```python
from build123d import *

# Parameters (mm, degrees)
SKETCH_1_W          = 70
SKETCH_1_H          = 70
EXTRUDE_1_DEPTH     = 3
CHAMFER_1_SIZE      = 6
SKETCH_2_R          = 2.1
CUT_EXTRUDE_1_DEPTH = 50.588305073
SKETCH_3_R          = 5.55
CUT_EXTRUDE_2_DEPTH = 50.588305073


with BuildPart() as part:
    # 草圖1 → 填料-伸長1 (new body)
    with BuildSketch(Plane.XY):
        Rectangle(SKETCH_1_W, SKETCH_1_H)
    extrude(amount=EXTRUDE_1_DEPTH)

    # 導角1
    chamfer_1_edges = [part.edges().sort_by_distance(p)[0] for p in [
        (-35, 35, 1.5),
        (35, 35, 1.5),
        (35, -35, 1.5),
        (-35, -35, 1.5),
    ]]
    chamfer(chamfer_1_edges, length=CHAMFER_1_SIZE)

    # 草圖2 → 除料-伸長1 (cut, through all)
    with BuildSketch(Plane(origin=(0, 0, 0), x_dir=(-1, 0, 0), z_dir=(0, 0, -1))):
        with Locations((0, 30)):
            Circle(SKETCH_2_R)
        with Locations((-30, -25)):
            Circle(SKETCH_2_R)
        with Locations((30, -25)):
            Circle(SKETCH_2_R)
    extrude(amount=-CUT_EXTRUDE_1_DEPTH, mode=Mode.SUBTRACT)

    # 草圖3 → 除料-伸長2 (cut, through all)
    with BuildSketch(Plane(origin=(0, 0, 0), x_dir=(-1, 0, 0), z_dir=(0, 0, -1))):
        with Locations((-17, 15)):
            Circle(SKETCH_3_R)
    extrude(amount=-CUT_EXTRUDE_2_DEPTH, mode=Mode.SUBTRACT)


solid = part.part
```
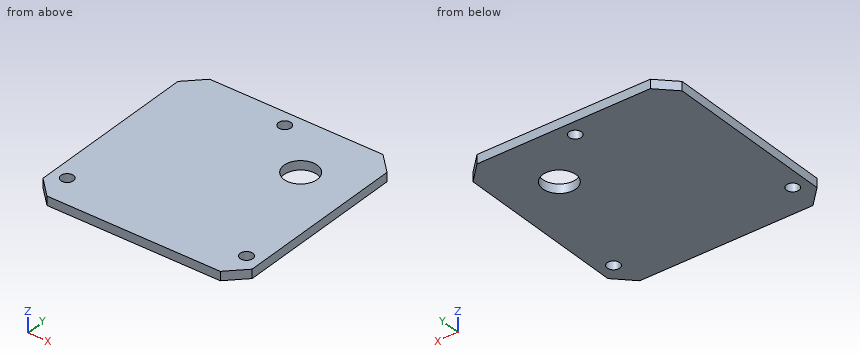
For this review, take the finished solid that the model builds, in its own axes (mm). Give positions to 0.01 mm unless a question says otherwise; leave off trailing zeros. Order: outer loops, then holes, each group sorted by start corner. A loop starts at its lowest first (then second) coordinate and runs counter-clockwise, first axis right, second up.
1) Wall thickness on line 1 (Y direction, x = 0, z = 1.1); line 2 (X direction, y = -24.5, z = 2.9); line 3 (X direction, y = 11.5, z = 0.6): over which ranges is each line inside the solid? List them lowest first.
2) Take a section at C-C (y = -25). Give the boundary of the cut face in (x, z), then the cut area to 3 significant figures.
3) Take a section at D-D (z = 2.3). Give the boundary of the cut face in (x, y), then the cut area to 3 significant figures.
4) Insertion check: pin 1 (6.5 mm diameter, centred on x = -30, y = -25, fed in from -Z); pin 2 (9 mm diameter, centred on x = 17, y = 15, fed in from +Z). Each pin has a flat end and moves straight along its axis. Give the tip position at first contact, or say it passes through.
5) Take a section at A-A (x = 0). Give the boundary of the cut face in (y, z).
6) Take a section at B-B (y = 15). Give the boundary of the cut face in (x, z), then the cut area to 3 significant figures.
Derived:
1. line 1: y = -35 to 27.9, 32.1 to 35
1. line 2: x = -35 to -32.04, -27.96 to 27.96, 32.04 to 35
1. line 3: x = -35 to 12.69, 21.31 to 35
2. outline: (-35, 0) - (-32.1, 0) - (-32.1, 3) - (-35, 3) - close; (-27.9, 0) - (27.9, 0) - (27.9, 3) - (-27.9, 3) - close; (32.1, 0) - (35, 0) - (35, 3) - (32.1, 3) - close
2. area: 185 mm2
3. outline: (-35, -29) - (-29, -35) - (29, -35) - (35, -29) - (35, 29) - (29, 35) - (-29, 35) - (-35, 29) - close; hole circle Ø4.2 at (-30, -25); hole circle Ø4.2 at (0, 30); hole circle Ø11.1 at (17, 15); hole circle Ø4.2 at (30, -25)
3. area: 4,690 mm2
4. pin 1: stops at z = 0
4. pin 2: passes through
5. outline: (-35, 0) - (27.9, 0) - (27.9, 3) - (-35, 3) - close; (32.1, 0) - (35, 0) - (35, 3) - (32.1, 3) - close
6. outline: (-35, 0) - (11.45, 0) - (11.45, 3) - (-35, 3) - close; (22.55, 0) - (35, 0) - (35, 3) - (22.55, 3) - close
6. area: 177 mm2
